Verification items for the finished model (mm, model axes). A direction names the side the tool comes from. Give positions to 0.01 mm unless a question says otherwise; leave off trailing zeros. Loops run counter-clockwise (first coordinate to the right, second up) from the corner with the lowest first, then second, coordinate; pieces in that order, holes last. Notation, with made-up numbers: M 42.5,-40 L 89.5,-40 A10 ccw 89.5,-31 Z; hole C 73.25,25 d8. An arc over 180 degrees is marked long. Answer in a Markdown table with one row per item.
```python
from build123d import *

# Parameters (mm, degrees)
CUT_EXTRUDE1_DEPTH      = 92.214667403
CUT_EXTRUDE1_DEPTH_BACK = 5
SKETCH2_R               = 1.5
CUT_EXTRUDE2_START      = 12
SKETCH3_R               = 4
CUT_EXTRUDE2_DEPTH      = 18


with BuildPart() as part:
    # Sketch1 → Revolve1 (revolve)
    with BuildSketch(Plane(origin=(0, 0, 0), x_dir=(1, 0, 0), z_dir=(0, 1, 0))):
        with BuildLine():
            Line((4.35, 0), (7.110769231, 0))
            Line((7.110769231, 0), (7.110769231, 7.110769231))
            Line((7.110769231, 7.110769231), (13, 13))
            Line((13, 13), (13, 25.966153846))
            Line((13, 25.966153846), (9.992154427, 28.973999419))
            ThreePointArc((9.992154427, 28.973999419), (7.439328335, 33.328329089), (7.33839208, 38.374805068))
            ThreePointArc((7.33839208, 38.374805068), (9.995816712, 63.953544784), (5.906153846, 89.342685943))
            Line((5.906153846, 89.342685943), (0, 89.342685943))
            Line((0, 89.342685943), (0, 24.5))
            Line((0, 24.5), (4.35, 24.5))
            Line((4.35, 24.5), (4.35, 0))
        make_face()
    revolve(axis=Axis((0, 0, 0), (0, 0, -1)))

    # Sketch2 → Cut-Extrude1 (cut, two sides: drawn at the far end of the back side and taken through both)
    with BuildSketch(Plane(origin=(0, 0, 0), x_dir=(1, 0, 0), z_dir=(0, 1, 0)).offset(-CUT_EXTRUDE1_DEPTH_BACK)):
        with Locations(Location((3.8, 18.5, 0), (0, 0, 270))):
            Circle(SKETCH2_R)
    extrude(amount=CUT_EXTRUDE1_DEPTH + CUT_EXTRUDE1_DEPTH_BACK, mode=Mode.SUBTRACT)

    # Sketch3 → Cut-Extrude2 (cut)
    with BuildSketch(Plane(origin=(0, -5, 0), x_dir=(1, 0, 0), z_dir=(0, 1, 0)).offset(CUT_EXTRUDE2_START)):
        with Locations(Location((3.8, 18.5, 0), (0, 0, 90))):
            Circle(SKETCH3_R)
    extrude(amount=CUT_EXTRUDE2_DEPTH, mode=Mode.SUBTRACT)


solid = part.part
```
Item 1: Sectioned sample at A-A (z = -18.5). Record the cut outline in (x, y).
Reported:
| item | result |
|---|---|
| outline | M -0.2,7 L -0.2,13 A13 ccw long 7.8,10.4 L 7.8,7 L 5.3,7 L 5.3,-5 L 2.3,-5 L 2.3,-3.69 A4.35 cw long 2.3,3.69 L 2.3,7 Z |
Item 2: Scan lines: L1, parallel to X at y = 0, z = -13; L2, parallel to Z at x = 3.8, y = -2.5; L3, parallel to Y at x = 0, z = -19.25. Record each from-to range of solid material in increasing order. Write a range as [from, to].
Reported:
| item | result |
|---|---|
| L1 | x = [-13, -4.35], [4.35, 13] |
| L2 | z = [-89.34, -20], [-17, 0] |
| L3 | y = [-13, -4.35], [4.35, 7] |
Item 3: Release check for a two-part mould opening along Y. For faces 1 (the flat face through (-3.1, -3.3, 0)), 2 (the cylindrical face through (-5.64, 4.33, -3.61)), 3 (the cylindrical face through (-4.346, -0.191, -12.078)), 4 (the flat face through (6, 7, -18)) record: released by +Y, released by -Y, zero draft, split by the parting line, or undercut.
Reported:
| item | result |
|---|---|
| face 1 | zero draft |
| face 2 | split by the parting line |
| face 3 | undercut |
| face 4 | released by +Y |
Item 4: Tool access check on faces 5 (the flat face through (0, 0, -89.343)), 6 (the flat face through (4, -5, -19)), 7 (the flat face through (0, 0, -24.5)). Record the directions out of +Z, -Z, +X, -X, +Y, -Y that give a thin tool (end or side, any length) a straight path to the whole face; none if there is none.
Reported:
| item | result |
|---|---|
| face 5 | -Z, +X, -X, +Y, -Y |
| face 6 | +Y |
| face 7 | +Z |
Item 5: Go/stop test with flat-tipped pins: pin 1 (6.5 mm diameter, centred on x = 3.5, z = -16.5, fed in from +Y); pin 2 (4 mm diameter, centred on x = 3.8, z = -18.5, fed in from +Y); pin 3 (5 mm diameter, centred on y = 6.5, z = -54.5, fed in from +X). Record where each tip stops, or that it passes through.
Reported:
| item | result |
|---|---|
| pin 1 | stops at y = 13 |
| pin 2 | stops at y = 7 |
| pin 3 | stops at x = 8.97 |
